```python
from build123d import *

# Parameters (mm, degrees)
SKETCH1_W           = 80
SKETCH1_H           = 5
BOSS_EXTRUDE1_DEPTH = 3
SKETCH2_R           = 1
CUT_EXTRUDE1_DEPTH  = 41.190172928
FILLET1_R           = 1


with BuildPart() as part:
    # Sketch1 → Boss-Extrude1 (new body)
    with BuildSketch(Plane.XY):
        Rectangle(SKETCH1_W, SKETCH1_H)
    extrude(amount=BOSS_EXTRUDE1_DEPTH)

    # Sketch2 → Cut-Extrude1 (cut, through all)
    with BuildSketch(Plane.XY.offset(3)):
        with Locations((-35, 0)):
            Circle(SKETCH2_R)
    extrude(amount=-CUT_EXTRUDE1_DEPTH, mode=Mode.SUBTRACT)

    # Fillet1
    fillet1_edges = [part.edges().sort_by_distance(p)[0] for p in [
        (-40, 2.5, 1.5),
        (40, 2.5, 1.5),
        (40, -2.5, 1.5),
        (-40, -2.5, 1.5),
    ]]
    fillet(fillet1_edges, radius=FILLET1_R)


solid = part.part
```
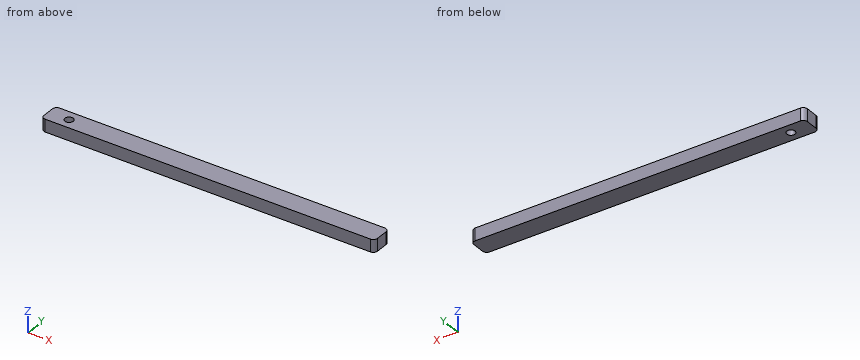
Work out the finished part from the listing and answer in its coordinate system (mm). Round coordinates to 2 decimals unless told otherwise and drop trailing zeros. Loops run counter-clockwise (first coordinate to the right, second up) from the corner with the lowest first, then second, coordinate; pieces in that order, holes last. Notation, with made-up numbers: M -21.75,86.5 L 29.25,86.5 A11 cw 29.25,105.5 Z; hole C 29,-7 d5. An arc over 180 degrees is marked long. Use CSV: the item, a comma, the result in double quotes.
Q1. Section A-A, the plane x = -35 is taken. Determine the outline of the cut face in (y, z), then the cut area to 3 significant figures.
Determined:
outline,"M -2.5,0 L -1,0 L -1,3 L -2.5,3 Z; M 1,0 L 2.5,0 L 2.5,3 L 1,3 Z"
area,"9.00 mm2"
Q2. Section B-B, the plane y = 0 is taken. Determine the outline of the cut face in (x, z).
Determined:
outline,"M -40,0 L -36,0 L -36,3 L -40,3 Z; M -34,0 L 40,0 L 40,3 L -34,3 Z"
Q3. This flat-tipped pin is pushed along its axis until it touches: pin 1 (1 mm diameter, centred on x = 31, y = -1.5, fed in from -Z). Where does it stop, or does it pass through?
Determined:
pin 1,"z = 0"
Q4. Consider L1, parallel to X at y = 0.15, z = 2.15; L2, parallel to Y at x = -35, z = 0.85; L3, parallel to X at y = -1.55, z = 1.8. Determine where each line is inside the solid, lowest interval first.
Determined:
L1,"-40 to -35.99, -34.01 to 40"
L2,"-2.5 to -1, 1 to 2.5"
L3,"-40 to 40"
